from build123d import *

# Parameters (mm, degrees)
SKETCH1_W            = 7.6
SKETCH1_H            = 9.6
BOSS_EXTRUDE1_DEPTH  = 15.8
SKETCH2_R            = 2.4
BOSS_EXTRUDE2_DEPTH  = 1.6
LPATTERN1_COUNT      = 2
LPATTERN1_PITCH      = 8
LPATTERN1_COUNT_DIR2 = 4
LPATTERN1_PITCH_DIR2 = 8
SHELL1_T             = -1.2


with BuildPart() as part:
    # Sketch1 → Boss-Extrude1 (new body)
    with BuildSketch(Plane.XY):
        with Locations((3.8, 4.8)):
            Rectangle(SKETCH1_W, SKETCH1_H)
    extrude(amount=-BOSS_EXTRUDE1_DEPTH)

    # Sketch2 → Boss-Extrude2 (add)
    with BuildSketch(Plane(origin=(0, 9.6, 0), x_dir=(1, 0, 0), z_dir=(0, 1, 0))):
        with Locations(Location((3.9, 3.9, 0), (0, 0, 270))):
            Circle(SKETCH2_R)
    boss_extrude2 = extrude(amount=BOSS_EXTRUDE2_DEPTH)

    # LPattern1: Boss-Extrude2 2 × 4, 6 skipped
    with Locations(*[(-j * LPATTERN1_PITCH_DIR2, 0, -i * LPATTERN1_PITCH) for i in range(LPATTERN1_COUNT) for j in range(LPATTERN1_COUNT_DIR2) if (i, j) not in ((0, 0), (0, 1), (0, 2), (0, 3), (1, 1), (1, 2), (1, 3))]):
        add(boss_extrude2)

    # Shell1
    shell1_openings = [part.faces().sort_by_distance(p)[0] for p in [
        (3.8, 0, -7.9),
    ]]
    offset(amount=SHELL1_T, openings=shell1_openings, kind=Kind.INTERSECTION)


solid = part.part
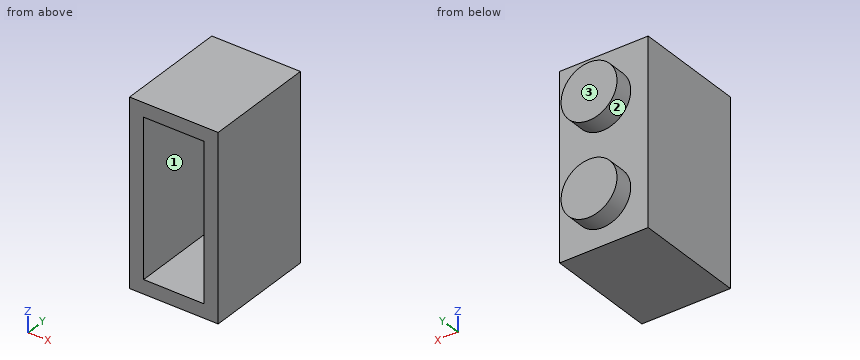
Input: part model. Units: mm. Frame: model coordinates. Face numbers are marked on the shaded views. A direction names the side the tool comes from. Round coordinates to 2 decimals unless told otherwise and drop trailing zeros. Order: outer loops, then holes, each group sorted by start corner. A loop starts at its lowest first (then second) coordinate and runs counter-clockwise, first axis right, second up. Notation, with made-up numbers: (27.5, -18.5) - (74.5, -18.5) arc R16 ccw to (74.5, 1.5) - close; hole circle Ø6 at (-13.75, 18). An arc over 180 degrees is marked (long way). Answer as a JSON object with one key per item and string values. Group by question number.
(1) Pin query (flat end, axial travel): P1, Ø1.2, axis at x = 4, z = -3.5, coming from the -Y side; P2, Ø1.5, axis at x = 6.5, z = -7, coming from the +Y side. Return the tip coordinate at first contact, or that it passes through.
(2) Cut plane A-A (y = 3). Return loops of the section in (x, z), then the cut area to 3 significant figures.
(3) Material intervals for probe 1 along Z at (x, y) = (3.9, 8.85); probe 2 along Z at (x, y) = (1.5, 6); probe 3 along X at (y, z) = (9.05, -11.9), sorted ascending. Write a range as from..to.
(4) Cut plane B-B (z = -3.9). Return loops of the section in (x, y).
(5) Reachability of the marked faces 1, 2 and 3 from +Z, -Z, +X, -X, +Y, -Y: full face, straight path, thin tool, end or side. Return the list, or none.
(6) Cut plane D-D (z = -8). Return loops of the section in (x, y).
(7) Cut plane C-C (x = 3.9). Return loops of the section in (y, z).
Here are the results:
{
 "1": {"P1": "stops at y = 10", "P2": "stops at y = 9.6"},
 "2": {"outline": "(0, -15.8) - (7.6, -15.8) - (7.6, 0) - (0, 0) - close; hole (1.2, -14.6) - (6.4, -14.6) - (6.4, -1.2) - (1.2, -1.2) - close", "area": "50.4 mm^2"},
 "3": {"probe 1": "z = -15.8..-13.1, -10.7..-5.1, -2.7..0", "probe 2": "z = -15.8..-14.6, -1.2..0", "probe 3": "x = 0..2.7, 5.1..7.6"},
 "4": {"outline": "(0, 0) - (1.2, 0) - (1.2, 8.4) - (2.7, 8.4) - (2.7, 10) - (5.1, 10) - (5.1, 8.4) - (6.4, 8.4) - (6.4, 0) - (7.6, 0) - (7.6, 9.6) - (6.3, 9.6) - (6.3, 11.2) - (1.5, 11.2) - (1.5, 9.6) - (0, 9.6) - close"},
 "5": {"face 1": "-Y", "face 2": "+Y", "face 3": "+Z, -Z, +X, -X, +Y"},
 "6": {"outline": "(0, 0) - (1.2, 0) - (1.2, 8.4) - (6.4, 8.4) - (6.4, 0) - (7.6, 0) - (7.6, 9.6) - (0, 9.6) - close"},
 "7": {"outline": "(0, -15.8) - (9.6, -15.8) - (9.6, -14.3) - (11.2, -14.3) - (11.2, -9.5) - (9.6, -9.5) - (9.6, -6.3) - (11.2, -6.3) - (11.2, -1.5) - (9.6, -1.5) - (9.6, 0) - (0, 0) - (0, -1.2) - (8.4, -1.2) - (8.4, -2.7) - (10, -2.7) - (10, -5.1) - (8.4, -5.1) - (8.4, -10.7) - (10, -10.7) - (10, -13.1) - (8.4, -13.1) - (8.4, -14.6) - (0, -14.6) - close"}
}
